The figure shows three views and two pictorial views of one solid part (mm, origin at its lowest corner). Answer the questions. A direction names the side the tool comes from. Coordinates: 2 decimals unless noted, no trailing zeros. Write each loop counter-clockwise with the first axis right and the second up, starting at its lowest first coordinate (ties: lowest second). Pieces come first, ordered by that corner, then holes.
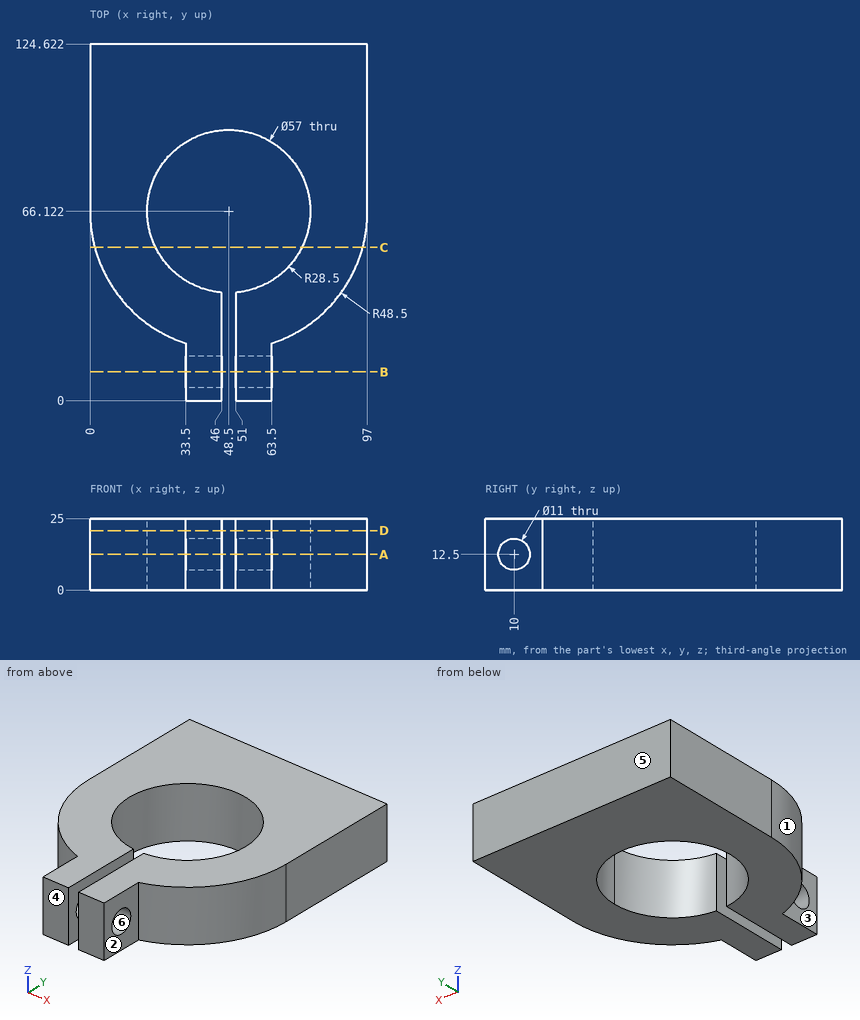
Q1. Find the intervals of material crossed by probe 1 along Z at (x, y) = (60.5, 10); probe 2 along X at (y, z) = (71.5, 17); probe 3 along X at (y, z) = (24, 6.5), in increasing order.
Answers below:
probe 1: z = 0 to 7, 18 to 25
probe 2: x = 0 to 20.51, 76.49 to 97
probe 3: x = 24.46 to 46, 51 to 72.54
Q2. The part is cut by section C-C, the plane y = 53.5. Write down the section's boundary in (x, z).
Answers below:
outline: (1.67, 0) - (22.95, 0) - (22.95, 25) - (1.67, 25) - close; (74.05, 0) - (95.33, 0) - (95.33, 25) - (74.05, 25) - close
Q3. The part is cut by section A-A, the plane z = 12.5. Write down the section's boundary in (x, y), then the cut area to 3 significant figures.
Answers below:
outline: (0, 66.12) arc R48.5 ccw to (33.5, 20) - (33.5, 15.5) - (46, 15.5) - (46, 37.73) arc R28.5 cw (long way) to (51, 37.73) - (51, 15.5) - (63.5, 15.5) - (63.5, 20) arc R48.5 ccw to (97, 66.12) - (97, 124.62) - (0, 124.62) - close; (33.5, 0) - (46, 0) - (46, 4.5) - (33.5, 4.5) - close; (51, 0) - (63.5, 0) - (63.5, 4.5) - (51, 4.5) - close
area: 6,910 mm2
Q4. Which of the six approach directions +Z, -Z, +X, -X, +Y, -Y give full straight-line access (tool end or side, diameter ignored) to the marked faces 1 and 2?
Answers below:
face 1: +Z, -Z, -X, -Y
face 2: +Z, -Z, +X, -Y
Q5. Determine the mould class of the marked faces 3, 4, 5 and 6 for opening direction Y: released by +Y, released by -Y, zero draft, split by the parting line, or undercut.
Answers below:
face 3: zero draft
face 4: released by -Y
face 5: released by +Y
face 6: undercut
Q6. The part is cut by section D-D, the plane z = 20.75. Write down the section's boundary in (x, y), then the cut area to 3 significant figures.
Answers below:
outline: (0, 66.12) arc R48.5 ccw to (33.5, 20) - (33.5, 0) - (46, 0) - (46, 37.73) arc R28.5 cw (long way) to (51, 37.73) - (51, 0) - (63.5, 0) - (63.5, 20) arc R48.5 ccw to (97, 66.12) - (97, 124.62) - (0, 124.62) - close
area: 7,180 mm2
Q7. The part is cut by section B-B, the plane y = 10. Write down the section's boundary in (x, z).
Answers below:
outline: (33.5, 0) - (46, 0) - (46, 7) - (33.5, 7) - close; (33.5, 18) - (46, 18) - (46, 25) - (33.5, 25) - close; (51, 0) - (63.5, 0) - (63.5, 7) - (51, 7) - close; (51, 18) - (63.5, 18) - (63.5, 25) - (51, 25) - close
Q8. Given pin 1 (1.5 mm diameter, centred on y = 40.5, z = 3, fed in from -X); pin 2 (7.5 mm diameter, centred on y = 21, z = 9, fed in from -X); pin 3 (3 mm diameter, centred on y = 17.5, z = 5, fed in from +X); pin 4 (6 mm diameter, centred on y = 9.5, z = 13, fed in from -X), each flat-ended and moving along its own axis, determine where each tip first touches the part or whether it passes through.
Answers below:
pin 1: stops at x = 6.86
pin 2: stops at x = 23.19
pin 3: stops at x = 63.5
pin 4: passes through
